The model under review builds one solid part; all positions refer to its coordinate system, in mm. Face numbers are marked on the shaded views. Coordinates: 2 decimals unless noted, no trailing zeros. Loops run counter-clockwise (first coordinate to the right, second up) from the corner with the lowest first, then second, coordinate; pieces in that order, holes last. Notation, with made-up numbers: M -6.75,3 L 0.25,3 A23 ccw 0.25,41 Z; hole C -14.5,19 d11. An arc over 180 degrees is marked long. Return JSON: item names as keys, results as strings.
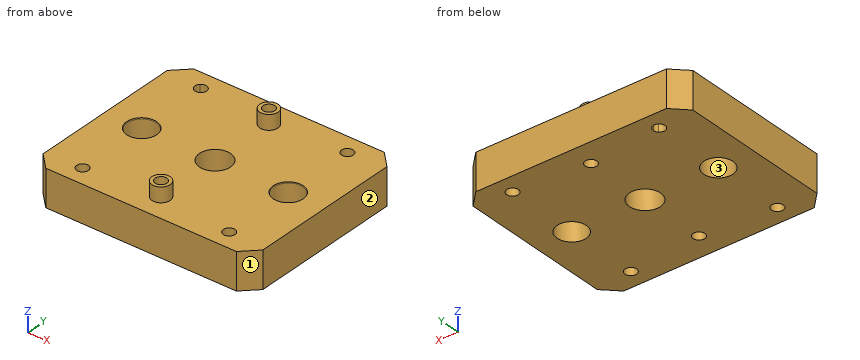
```python
from build123d import *

# Parameters (mm, degrees)
SKETCH_1_W                = 60
SKETCH_1_H                = 50
EXTRUDE_1_DEPTH           = 10
HOLE_WIZARD_1_D           = 8.5
HOLE_WIZARD_1_DEPTH       = 20
HOLE_WIZARD_2_D           = 8
HOLE_WIZARD_2_CSINK_D     = 8.2
HOLE_WIZARD_2_CSINK_ANGLE = 45
SKETCH_9_R                = 2.5
EXTRUDE_3_DEPTH           = 4
HOLE_WIZARD_3_D           = 3.2
CHAMFER_1_SIZE            = 4
SKETCH_15_R               = 1.6
CUT_EXTRUDE_1_DEPTH       = 41.311288741


with BuildPart() as part:
    # 草图1 → 凸台-拉伸1 (new body)
    with BuildSketch(Plane.XY):
        Rectangle(SKETCH_1_W, SKETCH_1_H)
    extrude(amount=EXTRUDE_1_DEPTH)

    # 孔1
    with Locations(Plane.XY.offset(10)):
        with Locations((0, 0)):
            Hole(HOLE_WIZARD_1_D / 2, depth=HOLE_WIZARD_1_DEPTH)

    # 孔2 (through all)
    with Locations(Plane.XY.offset(10)):
        with Locations((20, 0), (-20, 0)):
            CounterSinkHole(HOLE_WIZARD_2_D / 2, HOLE_WIZARD_2_CSINK_D / 2, counter_sink_angle=HOLE_WIZARD_2_CSINK_ANGLE)

    # 草图9 → 凸台-拉伸3 (add)
    with BuildSketch(Plane.XY.offset(10)):
        with Locations(Location((0, 18.25, 0), (0, 0, 180))):
            Circle(SKETCH_9_R)
        with Locations(Location((0, -18.25, 0), (0, 0, 180))):
            Circle(SKETCH_9_R)
    extrude(amount=EXTRUDE_3_DEPTH)

    # 孔3 (through all)
    with Locations(Plane.XY.offset(14)):
        with Locations((0, 18.25), (0, -18.25)):
            Hole(HOLE_WIZARD_3_D / 2)

    # 倒角1
    chamfer_1_edges = [part.edges().sort_by_distance(p)[0] for p in [
        (30, -25, 5),
        (-30, -25, 5),
        (-30, 25, 5),
        (30, 25, 5),
    ]]
    chamfer(chamfer_1_edges, length=CHAMFER_1_SIZE)

    # 草图15 → 切除-拉伸1 (cut, through all)
    with BuildSketch(Plane.XY.offset(10)):
        with BuildLine():
            ThreePointArc((-21.13137085, 21.13137085), (-21.13137085, 18.86862915), (-18.86862915, 18.86862915))
            Line((-18.86862915, 18.86862915), (-21.13137085, 21.13137085))
        make_face()
        with BuildLine():
            Line((-21.13137085, 21.13137085), (-18.86862915, 18.86862915))
            ThreePointArc((-18.86862915, 18.86862915), (-18.521792748, 19.387706508), (-18.4, 20))
            ThreePointArc((-18.4, 20), (-19.387706508, 21.478207252), (-21.13137085, 21.13137085))
        make_face()
        with Locations((20, 20)):
            Circle(SKETCH_15_R)
        with Locations((20, -20)):
            Circle(SKETCH_15_R)
        with Locations(Location((-20, -20, 0), (0, 0, 180))):
            Circle(SKETCH_15_R)
    extrude(amount=-CUT_EXTRUDE_1_DEPTH, mode=Mode.SUBTRACT)


solid = part.part
```
1. Insertion check: pin 1 Ø4 at (x, y) = (-20, -20) entering from +Z. The pin has a flat end and moves straight along its axis. Give the tip position at first contact, or say it passes through.
Check values:
{"pin 1": "z = 10"}
2. Add section A-A on y = 0. Give the boundary of the cut face in (x, z).
Check values:
{"outline": "M -30,0 L -24,0 L -24,9.76 L -24.1,10 L -30,10 Z; M -16,0 L -4.25,0 L -4.25,10 L -15.9,10 L -16,9.76 Z; M 4.25,0 L 16,0 L 16,9.76 L 15.9,10 L 4.25,10 Z; M 24,0 L 30,0 L 30,10 L 24.1,10 L 24,9.76 Z"}
3. Add section C-C on z = 3. State how many separate pieces and enclosed holes the cut face has, plus the area to 3 significant figures.
Check values:
{"separate pieces": "1", "enclosed holes": "9", "area": "2,760 mm²"}
4. The part is to be moulded in two halves that separate along Y. For the marked faces 1, 2 and 3, say which applies: released by +Y, released by -Y, zero draft, split by the parting line, or undercut.
Check values:
{"face 1": "released by -Y", "face 2": "zero draft", "face 3": "undercut"}
5. To check wall thickness, follow line 1 (Y direction, x = 20, z = 6); line 2 (Y direction, x = 0, z = 11.25); line 3 (X direction, y = -19, z = 3.25). State the ranges of each line that lie inside material, in increasing order.
Check values:
{"line 1": "-25 to -21.6, -18.4 to -4, 4 to 18.4, 21.6 to 25", "line 2": "-20.75 to -19.85, -16.65 to -15.75, 15.75 to 16.65, 19.85 to 20.75", "line 3": "-30 to -21.25, -18.75 to -1.41, 1.41 to 18.75, 21.25 to 30"}
6. Add section D-D on x = 0. Give the boundary of the cut face in (y, z).
Check values:
{"outline": "M -25,0 L -19.85,0 L -19.85,14 L -20.75,14 L -20.75,10 L -25,10 Z; M -16.65,0 L -4.25,0 L -4.25,10 L -15.75,10 L -15.75,14 L -16.65,14 Z; M 4.25,0 L 16.65,0 L 16.65,14 L 15.75,14 L 15.75,10 L 4.25,10 Z; M 19.85,0 L 25,0 L 25,10 L 20.75,10 L 20.75,14 L 19.85,14 Z"}
7. Add section B-B on x = 20. Give the boundary of the cut face in (y, z), plus the area to 3 significant figures.
Check values:
{"outline": "M -25,0 L -21.6,0 L -21.6,10 L -25,10 Z; M -18.4,0 L -4,0 L -4,9.76 L -4.1,10 L -18.4,10 Z; M 4,0 L 18.4,0 L 18.4,10 L 4.1,10 L 4,9.76 Z; M 21.6,0 L 25,0 L 25,10 L 21.6,10 Z", "area": "356 mm²"}
